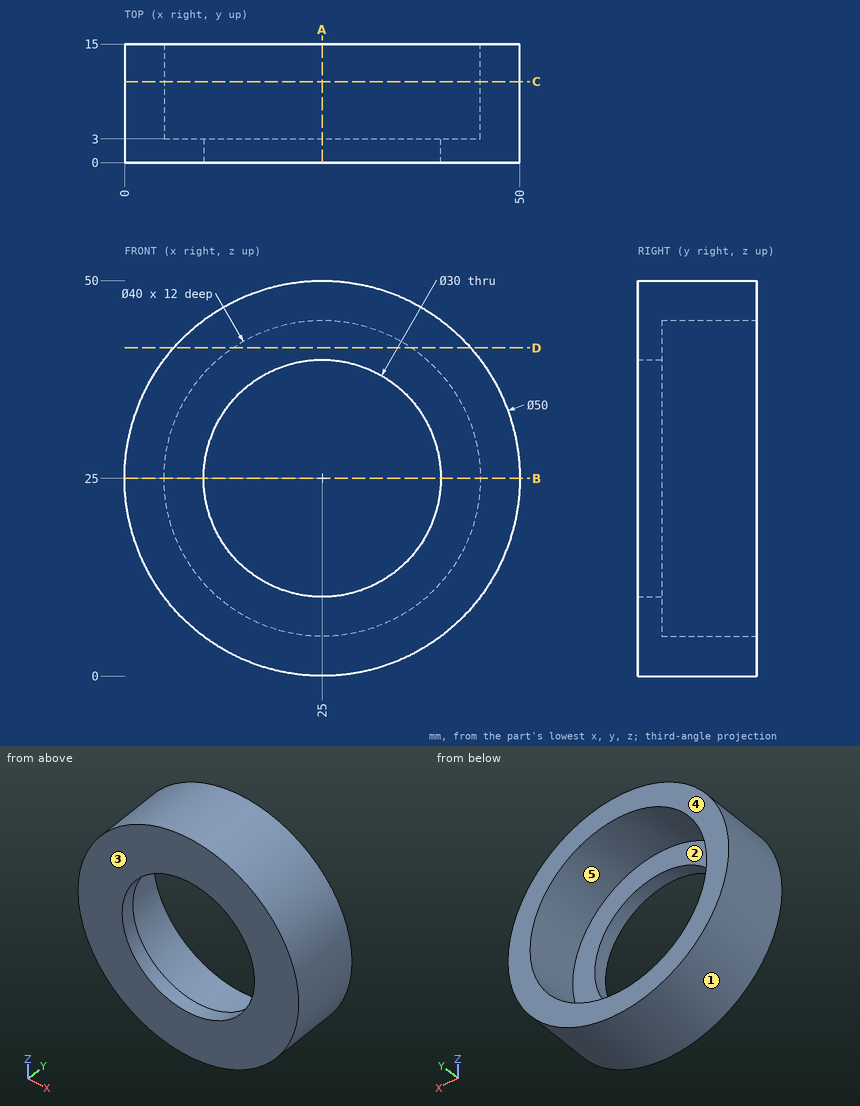
Design review of the part shown in the three views and the two pictorial views. Dimensions are in mm from the part's minimum x, y and z. A direction names the side the tool comes from. Give positions to 0.01 mm unless a question says otherwise; leave off trailing zeros. Order: outer loops, then holes, each group sorted by start corner. A loop starts at its lowest first (then second) coordinate and runs counter-clockwise, first axis right, second up. Notation, with made-up numbers: (52.25, 68.25) -> (81.25, 68.25) arc R18 ccw to (81.25, 100.25) -> close; hole circle Ø3 at (9.25, 21.5). An arc over 180 degrees is marked (long way). Write each question's results on one line, items separated by ' | '. Start each with the question number.
Q1. Wall thickness on L1, parallel to Z at x = 25, y = 12.25; L2, parallel to X at y = 6.5, z = 34; L3, parallel to X at y = 12.25, z = 40: over which ranges is each line inside the solid? List them lowest first. Write a range as from..to.
Q2. Add section B-B on z = 25. Give the boundary of the cut face in (x, y).
Q3. Add section D-D on z = 41.5. Give the boundary of the cut face in (x, y), and give its area (3 significant figures).
Q4. For pin 1 (1.5 mm diameter, centred on x = 31.5, y = 8.5, fed in from -Z); pin 2 (2 mm diameter, centred on y = 4, z = 9.5, fed in from +X); pin 3 (6 mm diameter, centred on y = 2.5, z = 38, fed in from +X), all flat-tipped, find the tip position at first contact; note any pin that passes through.
Q5. Add section C-C on y = 10.25. Give the boundary of the cut face in (x, z).
Q6. Machinability: for the marked faces 4 and 5, which of the approach directions +Z, -Z, +X, -X, +Y, -Y give a long, thin tool a straight path to every point of the face, cutting with its end or side? Answer none if there is none.
Q7. Add section A-A on x = 25. Give the boundary of the cut face in (y, z).
Q8. Mouldability with a two-part tool opening along X and no side actions: class the marked faces 1, 2 and 3 as +X half, -X half, draft (parallel to the pull), parting line (faces both ways), or undercut.
Found:
1) L1: z = 0..5, 45..50 | L2: x = 1.68..7.14, 42.86..48.32 | L3: x = 5..11.77, 38.23..45
2) outline: (0, 0) -> (10, 0) -> (10, 3) -> (5, 3) -> (5, 15) -> (0, 15) -> close; (40, 0) -> (50, 0) -> (50, 15) -> (45, 15) -> (45, 3) -> (40, 3) -> close
3) outline: (6.22, 0) -> (43.78, 0) -> (43.78, 15) -> (36.3, 15) -> (36.3, 3) -> (13.7, 3) -> (13.7, 15) -> (6.22, 15) -> close | area: 292 mm2
4) pin 1: stops at z = 0.67 | pin 2: stops at x = 45.37 | pin 3: stops at x = 47.91
5) outline: circle Ø50 at (25, 25); hole circle Ø40 at (25, 25)
6) face 4: +Z, -Z, +X, -X, +Y | face 5: +Y
7) outline: (0, 0) -> (15, 0) -> (15, 5) -> (3, 5) -> (3, 10) -> (0, 10) -> close; (0, 40) -> (3, 40) -> (3, 45) -> (15, 45) -> (15, 50) -> (0, 50) -> close
8) face 1: parting line | face 2: undercut | face 3: draft
